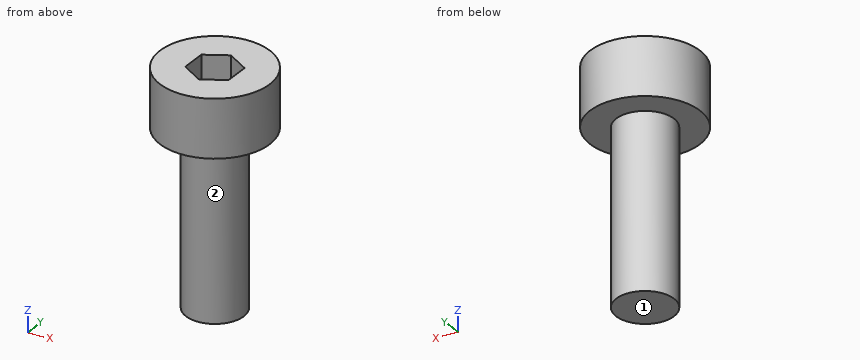
```python
from build123d import *

# Parameters (mm, degrees)
SKETCH_1_R          = 1.9
EXTRUDE_1_DEPTH     = 2
SKETCH_2_R          = 1
EXTRUDE_2_DEPTH     = 6
CUT_EXTRUDE_1_DEPTH = 1


with BuildPart() as part:
    # 草图1 → 凸台-拉伸1 (new body)
    with BuildSketch(Plane.XY):
        Circle(SKETCH_1_R)
    extrude(amount=EXTRUDE_1_DEPTH)

    # 草图2 → 凸台-拉伸2 (add)
    with BuildSketch(Plane(origin=(0, 0, 0), x_dir=(-1, 0, 0), z_dir=(0, 0, -1))):
        Circle(SKETCH_2_R)
    extrude(amount=EXTRUDE_2_DEPTH)

    # 草图3 → 切除-拉伸1 (cut)
    with BuildSketch(Plane.XY.offset(2)):
        Polygon((-0.766222709, -0.403612141), (-0.033572987, -0.865374401), (0.732649722, -0.461762261), (0.766222709, 0.403612141), (0.033572987, 0.865374401), (-0.732649722, 0.461762261), align=None)
    extrude(amount=-CUT_EXTRUDE_1_DEPTH, mode=Mode.SUBTRACT)


solid = part.part
```
Design review of the part built by this model. Coordinates are the model's own, in mm. Face numbers are marked on the shaded views. A direction names the side the tool comes from. Give positions to 0.01 mm unless a question says otherwise; leave off trailing zeros. Write each loop counter-clockwise with the first axis right and the second up, starting at its lowest first coordinate (ties: lowest second). Pieces come first, ordered by that corner, then holes.
(1) Add section A-A (z = 1.75). Give the boundary of the cut face in (x, y).
Checked values:
outline: circle Ø3.8 at (0, 0); hole (-0.77, -0.4) - (-0.03, -0.87) - (0.73, -0.46) - (0.77, 0.4) - (0.03, 0.87) - (-0.73, 0.46) - close
(2) Clearance check with flat-ended pins moving along their axes: pin 1 Ø1.5 at (y, z) = (1, -2.5) entering from +X; pin 2 Ø0.5 at (x, y) = (0, 0) entering from +Z; pin 3 Ø1 at (x, z) = (0.5, -4) entering from +Y. State where each tip first meets the part, or that it passes through.
Checked values:
pin 1: stops at x = 0.97
pin 2: stops at z = 1
pin 3: stops at y = 1
(3) Add section B-B (y = 0). Give the boundary of the cut face in (x, z).
Checked values:
outline: (-1.9, 0) - (-1, 0) - (-1, -6) - (1, -6) - (1, 0) - (1.9, 0) - (1.9, 2) - (0.75, 2) - (0.75, 1) - (-0.75, 1) - (-0.75, 2) - (-1.9, 2) - close
(4) Tool access review of the marked faces 1 and 2: name each direction out of +Z, -Z, +X, -X, +Y, -Y from which nothing blocks a thin tool from reaching the whole face with its end or side.
Checked values:
face 1: -Z, +X, -X, +Y, -Y
face 2: -Z
(5) Wall thickness on line 1 along Z through (x, y) = (-1.45, 0.4); line 2 along Z through (x, y) = (-0.65, -0.35); line 3 along Y through (x, z) = (-0.05, -3.5): over which ranges is each line inside the solid? List them lowest first.
Checked values:
line 1: z = 0 to 2
line 2: z = -6 to 1
line 3: y = -1 to 1
(6) Add section C-C (z = -1.75). Give the boundary of the cut face in (x, y), and give its area (3 significant figures).
Checked values:
outline: circle Ø2 at (0, 0)
area: 3.14 mm2
(7) Add section D-D (x = 0.35). Give the boundary of the cut face in (y, z).
Checked values:
outline: (-1.87, 0) - (-0.94, 0) - (-0.94, -6) - (0.94, -6) - (0.94, 0) - (1.87, 0) - (1.87, 2) - (0.67, 2) - (0.67, 1) - (-0.66, 1) - (-0.66, 2) - (-1.87, 2) - close
